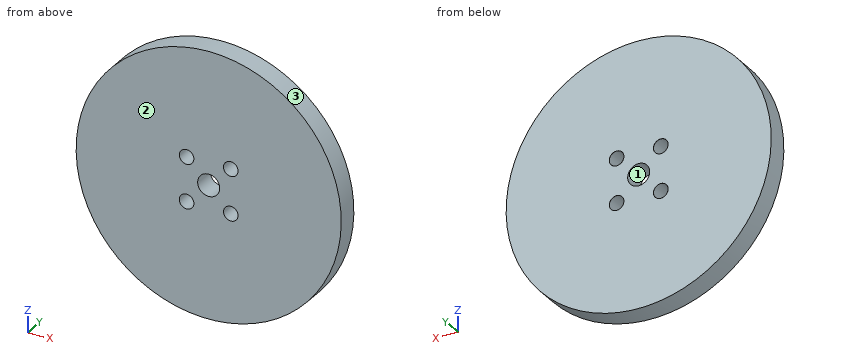
```python
from build123d import *

# Parameters (mm, degrees)
SKETCH1_R                      = 60
SKETCH1_R_2                    = 5
BOSS_EXTRUDE1_DEPTH            = 10
M6_CLEARANCE_HOLE1_D           = 6.6
M6_CLEARANCE_HOLE1_CSINK_D     = 6.65
M6_CLEARANCE_HOLE1_CSINK_ANGLE = 100


with BuildPart() as part:
    # Sketch1 → Boss-Extrude1 (new body)
    with BuildSketch(Plane(origin=(0, 0, 0), x_dir=(1, 0, 0), z_dir=(0, 1, 0))):
        with Locations(Location((0, 0, 0), (0, 0, 270))):
            Circle(SKETCH1_R)
        with Locations(Location((0, 0, 0), (0, 0, 270))):
            Circle(SKETCH1_R_2, mode=Mode.SUBTRACT)
    extrude(amount=BOSS_EXTRUDE1_DEPTH)

    # M6 Clearance Hole1 (through all)
    with Locations(Plane(origin=(0, 10, 0), x_dir=(1, 0, 0), z_dir=(0, 1, 0))):
        with Locations((-10, 10), (10, 10), (-10, -10), (10, -10)):
            CounterSinkHole(M6_CLEARANCE_HOLE1_D / 2, M6_CLEARANCE_HOLE1_CSINK_D / 2, counter_sink_angle=M6_CLEARANCE_HOLE1_CSINK_ANGLE)


solid = part.part
```
Geometry check sheet. Reference: the model listing, model coordinates, mm. Face numbers are marked on the shaded views. Round coordinates to 2 decimals unless told otherwise and drop trailing zeros. Loops run counter-clockwise (first coordinate to the right, second up) from the corner with the lowest first, then second, coordinate; pieces in that order, holes last. Notation, with made-up numbers: (27, 49.5) -> (57, 49.5) arc R23 cw to (57, 66.5) -> close; hole circle Ø6 at (49, 36.25). An arc over 180 degrees is marked (long way). Use a Markdown table: item, result.
(1) Sectioned sample at B-B (x = -10). Enter the section's corners in (y, z) (3 decimals).
Calculated:
| item | result |
|---|---|
| outline | (0, -59.161) -> (10, -59.161) -> (10, -13.325) -> (9.979, -13.3) -> (0, -13.3) -> close; (0, -6.7) -> (9.979, -6.7) -> (10, -6.675) -> (10, 6.675) -> (9.979, 6.7) -> (0, 6.7) -> close; (0, 13.3) -> (9.979, 13.3) -> (10, 13.325) -> (10, 59.161) -> (0, 59.161) -> close |
(2) Sectioned sample at C-C (y = 2). Enter the section's corners in (x, z).
Calculated:
| item | result |
|---|---|
| outline | circle Ø120 at (0, 0); hole circle Ø6.6 at (-10, -10); hole circle Ø6.6 at (-10, 10); hole circle Ø10 at (0, 0); hole circle Ø6.6 at (10, -10); hole circle Ø6.6 at (10, 10) |
(3) Sectioned sample at D-D (x = -22.5). Enter the section's corners in (y, z), then the cut area to 3 significant figures.
Calculated:
| item | result |
|---|---|
| outline | (0, -55.62) -> (10, -55.62) -> (10, 55.62) -> (0, 55.62) -> close |
| area | 1,110 mm² |
(4) Mould release check, pull along X, two halves, no side actions. Record for the marked faces 1, 2 and 3: released by +X, released by -X, zero draft, split by the parting line, or undercut.
Calculated:
| item | result |
|---|---|
| face 1 | undercut |
| face 2 | zero draft |
| face 3 | split by the parting line |
(5) Sectioned sample at A-A (z = 0). Enter the section's corners in (x, y).
Calculated:
| item | result |
|---|---|
| outline | (-60, 0) -> (-5, 0) -> (-5, 10) -> (-60, 10) -> close; (5, 0) -> (60, 0) -> (60, 10) -> (5, 10) -> close |
(6) Scan lines: probe 1 along X at (y, z) = (2.5, 0); probe 2 along X at (y, z) = (3.75, 10). Record each from-to range of solid material in increasing order.
Calculated:
| item | result |
|---|---|
| probe 1 | -60 to -5, 5 to 60 |
| probe 2 | -59.16 to -13.3, -6.7 to 6.7, 13.3 to 59.16 |
(7) Go/stop test with flat-tipped pins: P1, Ø1, axis at y = 3, z = 5.5, coming from the -X side; P2, Ø1, axis at y = 2, z = 39.5, coming from the +X side; P3, Ø1.5, axis at x = 27, y = 4, coming from the -Z side. Record where each tip stops, or that it passes through.
Calculated:
| item | result |
|---|---|
| P1 | x = -59.79 |
| P2 | x = 45.6 |
| P3 | z = -53.95 |
